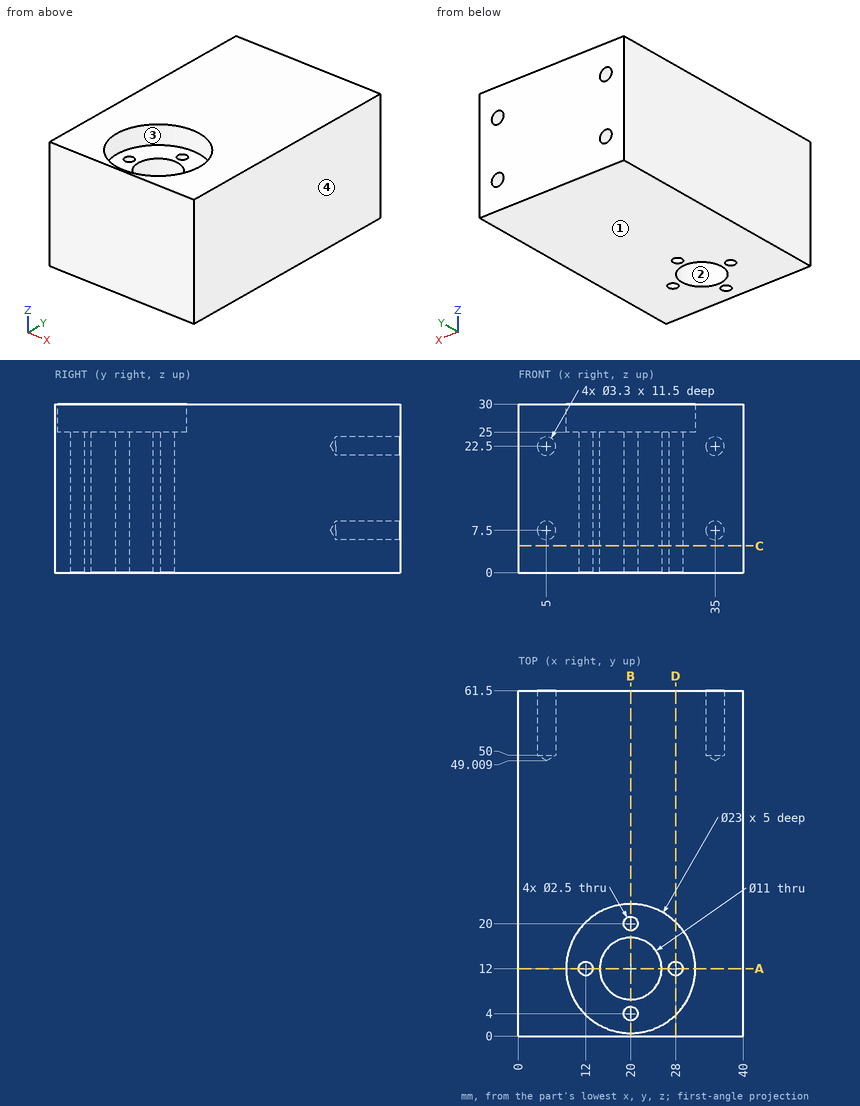
The drawing under review shows one solid part. Ordinate dimensions are in mm from its lowest x, y, z. Coordinates: 2 decimals unless noted, no trailing zeros. Loops run counter-clockwise (first coordinate to the right, second up) from the corner with the lowest first, then second, coordinate; pieces in that order, holes last. Notation, with made-up numbers: M 44.5,-5 L 98.5,-5 A28 ccw 98.5,31 Z; hole C -38,26.5 d9. An arc over 180 degrees is marked long. Use one line per item in the form item = value.
(1) Consider section A-A (y = 12). Write out the cut boundary in (x, z), and give its area (3 significant figures).
Return value:
outline = M 0,0 L 10.75,0 L 10.75,25 L 8.5,25 L 8.5,30 L 0,30 Z; M 13.25,0 L 14.5,0 L 14.5,25 L 13.25,25 Z; M 25.5,0 L 26.75,0 L 26.75,25 L 25.5,25 Z; M 29.25,0 L 40,0 L 40,30 L 31.5,30 L 31.5,25 L 29.25,25 Z
area = 685 mm2
(2) Consider section C-C (z = 4.75). Write out the cut boundary in (x, y).
Return value:
outline = M 0,0 L 40,0 L 40,61.5 L 0,61.5 Z; hole C 12,12 d2.5; hole C 20,12 d11; hole C 20,4 d2.5; hole C 20,20 d2.5; hole C 28,12 d2.5
(3) Consider section D-D (x = 28). Write out the cut boundary in (y, z).
Return value:
outline = M 0,0 L 10.75,0 L 10.75,25 L 3.74,25 L 3.74,30 L 0,30 Z; M 13.25,0 L 61.5,0 L 61.5,30 L 20.26,30 L 20.26,25 L 13.25,25 Z
(4) Draft analysis for pull direction X (two halves, no side actions). For the marked faces 1, 2, 3 and 4, state which applies: pulls with the +X half, pulls with the -X half, needs draft (parallel to the pull), parting line crosses it, or undercut.
Return value:
face_1 = needs draft
face_2 = undercut
face_3 = undercut
face_4 = pulls with the +X half
(5) Clearance check with flat-ended pins moving along their axes: P1, Ø3, axis at x = 20, y = 4, coming from the +Z side; P2, Ø2, axis at x = 35, z = 7.5, coming from the +Y side; P3, Ø3, axis at x = 5, z = 22.5, coming from the +Y side; P4, Ø2, axis at x = 12, y = 12, coming from the -Z side (1 decimal). State where each tip first meets the part, or that it passes through.
Return value:
P1 = 25
P2 = 49.61
P3 = 49.91
P4 = through
(6) Consider section B-B (x = 20). Write out the cut boundary in (y, z), and give its area (3 significant figures).
Return value:
outline = M 0,0 L 2.75,0 L 2.75,25 L 0.5,25 L 0.5,30 L 0,30 Z; M 5.25,0 L 6.5,0 L 6.5,25 L 5.25,25 Z; M 17.5,0 L 18.75,0 L 18.75,25 L 17.5,25 Z; M 21.25,0 L 61.5,0 L 61.5,30 L 23.5,30 L 23.5,25 L 21.25,25 Z
area = 1,330 mm2
(7) For line 1 along Y through (x, z) = (20, 10.25); line 2 along X through (y, z) = (53.5, 22.5); line 3 along Z through (x, y) = (36, 58.5), list the stretches that pass through material, from the lowest coordinate up. Write a range as from..to.
Return value:
line_1 = 0..2.75, 5.25..6.5, 17.5..18.75, 21.25..61.5
line_2 = 0..3.35, 6.65..33.35, 36.65..40
line_3 = 0..6.19, 8.81..21.19, 23.81..30
